Verification items for the finished model (mm, model axes). Round coordinates to 2 decimals unless told otherwise and drop trailing zeros. Order: outer loops, then holes, each group sorted by start corner. A loop starts at its lowest first (then second) coordinate and runs counter-clockwise, first axis right, second up. Notation, with made-up numbers: (56.5, -3) -> (73.5, -3) arc R15 ccw to (73.5, 2) -> close; hole circle Ø1 at (-31, -3). An arc over 180 degrees is marked (long way). Return JSON: item names as keys, results as strings. Group by question number.
1) Section check B-B on z = 9. Enter the section's corners in (x, y), plus the area to 3 significant figures.
2) Scan lines: L1, parallel to Y at x = 2.5, z = 4; L2, parallel to X at y = 2.65, z = 17.5; L3, parallel to X at y = 1.75, z = -5.5. Record each from-to range of solid material in increasing order.
3) Section check C-C on y = 2.35. Enter the section's corners in (x, z), plus the area to 3 significant figures.
4) Depth check by flat-ended pin: pin 1 (2 mm diameter, centred on x = 3.5, y = 4, fed in from +Z); pin 2 (1.2 mm diameter, centred on x = 16.5, z = 13, fed in from +Y); pin 3 (2.5 mm diameter, centred on x = 3.5, y = 3, fed in from -Z). Enter the tip coordinate at first touch or a pass-through.
5) Section check A-A on x = 2.5. Enter the section's corners in (y, z).
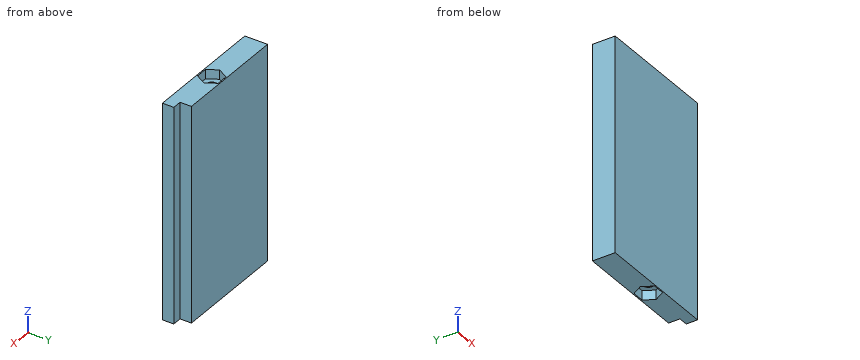
```python
from build123d import *

# Parameters (mm, degrees)
SKETCH1_W           = 30
SKETCH1_H           = 56.5
BOSS_EXTRUDE1_DEPTH = 6
SKETCH8_W           = 56.5
SKETCH8_H           = 3
BOSS_EXTRUDE3_DEPTH = 2.45
SKETCH9_R           = 1.5
CUT_EXTRUDE3_DEPTH  = 60.436962406
CUT_EXTRUDE4_DEPTH  = 2.45


with BuildPart() as part:
    # Sketch1 → Boss-Extrude1 (new body)
    with BuildSketch(Plane(origin=(0, 0, 0), x_dir=(1, 0, 0), z_dir=(0, 1, 0))):
        Rectangle(SKETCH1_W, SKETCH1_H)
    extrude(amount=BOSS_EXTRUDE1_DEPTH)

    # Sketch8 → Boss-Extrude3 (add)
    with BuildSketch(Plane(origin=(15, 0, 0), x_dir=(0, 0, -1), z_dir=(1, 0, 0))):
        with Locations((0, 1.5)):
            Rectangle(SKETCH8_W, SKETCH8_H)
    extrude(amount=BOSS_EXTRUDE3_DEPTH)

    # Sketch9 → Cut-Extrude3 (cut, through all)
    with BuildSketch(Plane(origin=(0, 0, -28.25), x_dir=(-1, 0, 0), z_dir=(0, 0, -1))):
        with Locations((-2.5, 3)):
            Circle(SKETCH9_R)
    extrude(amount=-CUT_EXTRUDE3_DEPTH, mode=Mode.SUBTRACT)

    # Sketch10 → Cut-Extrude4 (cut)
    with BuildSketch(Plane(origin=(0, 0, -28.25), x_dir=(-1, 0, 0), z_dir=(0, 0, -1))):
        Polygon((-0.941154273, 0.3), (0.617691454, 3), (-0.941154273, 5.7), (-4.058845727, 5.7), (-5.617691454, 3), (-4.058845727, 0.3), align=None)
    cut_extrude4 = extrude(amount=-CUT_EXTRUDE4_DEPTH, mode=Mode.SUBTRACT)

    # Mirror2: Cut-Extrude4 across plane
    add(cut_extrude4.mirror(Plane.XY), mode=Mode.SUBTRACT)


solid = part.part
```
Check result:
{
 "1": {"outline": "(-15, 0) -> (17.45, 0) -> (17.45, 3) -> (15, 3) -> (15, 6) -> (-15, 6) -> close; hole circle Ø3 at (2.5, 3)", "area": "180 mm^2"},
 "2": {"L1": "0 to 1.5, 4.5 to 6", "L2": "-15 to 1.04, 3.96 to 17.45", "L3": "-15 to 1.67, 3.33 to 17.45"},
 "3": {"outline": "(-15, -28.25) -> (-0.24, -28.25) -> (-0.24, -25.8) -> (1.15, -25.8) -> (1.15, 25.8) -> (-0.24, 25.8) -> (-0.24, 28.25) -> (-15, 28.25) -> close; (3.85, -25.8) -> (5.24, -25.8) -> (5.24, -28.25) -> (17.45, -28.25) -> (17.45, 28.25) -> (5.24, 28.25) -> (5.24, 25.8) -> (3.85, 25.8) -> close", "area": "1,670 mm^2"},
 "4": {"pin 1": "z = 25.8", "pin 2": "y = 3", "pin 3": "z = -25.8"},
 "5": {"outline": "(0, -28.25) -> (0.3, -28.25) -> (0.3, -25.8) -> (1.5, -25.8) -> (1.5, 25.8) -> (0.3, 25.8) -> (0.3, 28.25) -> (0, 28.25) -> close; (4.5, -25.8) -> (5.7, -25.8) -> (5.7, -28.25) -> (6, -28.25) -> (6, 28.25) -> (5.7, 28.25) -> (5.7, 25.8) -> (4.5, 25.8) -> close"}
}
